Build history of the part. All positions in model axes, mm. A direction names the side the tool comes from. Give positions to 0.01 mm unless a question says otherwise; leave off trailing zeros. Loops run counter-clockwise (first coordinate to the right, second up) from the corner with the lowest first, then second, coordinate; pieces in that order, holes last.
1) Band-saw the part on B-B on x = -0.7. List the corners of the cut face in (y, z), then the cut area to 3 significant figures.
2) Band-saw the part on A-A on z = 0. List the corners of the cut face in (x, y).
3) Band-saw the part on D-D on x = 1.5. List the corners of the cut face in (y, z), then the cut area to 3 significant figures.
4) Two-plate mould, pull along X, no slides. Class faces 5 (the cylindrical face through (1, 6, 0)), 6 (the flat face through (-1.299, 1, 0)), 7 (the flat face through (1, 12, 1)): +X half, -X half, draft (parallel to the pull), parting line (faces both ways), or undercut.
5) Flat gauge pins, fed straight in: P1, Ø1.5, axis at y = 6.5, z = 1.5, coming from the -X side; P2, Ø1.6, axis at y = 1, z = 0, coming from the -X side; P3, Ø1.2, axis at y = 0.5, z = 0.5, coming from the +X side. Where does each tip first touch, or does it go through?
6) 3-axis set-ups, long thin cutter, end or side, ignore diameter. For faces 1 (the flat face through (1.299, 1, 0)), 2 (the flat face through (0.64, 0.99, -1.13)), 3 (the flat face through (-0.66, 0.99, -1.12)), 4 (the flat face through (0.66, 0.99, 1.12)): which of +Z, -Z, +X, -X, +Y, -Y reach the whole face in a straight line?
7) Wall check: line 1 (Z direction, x = 0, y = 6.25); line 2 (Y direction, x = -2.2, z = -0.2). Give the ranges that are in metal, low to high.
8) Band-saw the part on C-C on y = 4.5. List the corners of the cut face in (x, z), then the cut area to 3 significant figures.
Autodesk Inventor part; units mm, degrees
ref_plane "YZ Plane" through (0, 0, 0) normal (1, 0, 0) x (0, 1, 0)
ref_plane "XZ Plane" through (0, 0, 0) normal (0, 1, 0) x (-1, 0, 0)
ref_plane "XY Plane" through (0, 0, 0) normal (0, 0, 1) x (1, 0, 0)
sketch "Sketch1" plane through (0, 0, 0) normal (0, 1, 0) x (-1, 0, 0)
  circle A0 centre (0, 0) radius 1.5 construction
  line L0 (0, -1.5) -> (-1.299, -0.75)
  line L1 (-1.299, -0.75) -> (-1.299, 0.75)
  line L2 (-1.299, 0.75) -> (0, 1.5)
  line L3 (0, 1.5) -> (1.299, 0.75)
  line L4 (1.299, 0.75) -> (1.299, -0.75)
  line L5 (1.299, -0.75) -> (0, -1.5)
  dimension "d0" = 3
extrude "Extrusion1" add sketch "Sketch1" along normal blind 2
sketch "Sketch2" plane through (0, 2, 0) normal (0, 1, 0) x (1, 0, 0)
  circle A0 centre (0, 0) radius 2.5
  dimension "d3" = 5
extrude "Extrusion2" add sketch "Sketch2" along normal blind 10
sketch "Sketch3" plane through (0, 12, 0) normal (0, 1, 0) x (1, 0, 0)
  circle A0 centre (0, 0) radius 2.5
hole "Hole1" at (0, 12, 0) direction (0, -1, 0) diameter 2 end through all
properties part number "separator" material "PET Plastic"
Findings below:
1. outline: (0, -1.1) - (2, -1.1) - (2, -2.4) - (12, -2.4) - (12, -0.71) - (0, -0.71) - close; (0, 0.71) - (12, 0.71) - (12, 2.4) - (2, 2.4) - (2, 1.1) - (0, 1.1) - close
1. area: 35.2 mm2
2. outline: (-2.5, 2) - (-1.3, 2) - (-1.3, 0) - (-1, 0) - (-1, 12) - (-2.5, 12) - close; (1, 0) - (1.3, 0) - (1.3, 2) - (2.5, 2) - (2.5, 12) - (1, 12) - close
3. outline: (2, -2) - (12, -2) - (12, 2) - (2, 2) - close
3. area: 40.0 mm2
4. face 5: undercut
4. face 6: -X half
4. face 7: draft
5. P1: stops at x = -2.38
5. P2: stops at x = -1.3
5. P3: stops at x = 1.3
6. face 1: +Z, -Z, +X, -Y
6. face 2: -Z, +X, -Y
6. face 3: -Z, -X, -Y
6. face 4: +Z, +X, -Y
7. line 1: z = -2.5 to -1, 1 to 2.5
7. line 2: y = 2 to 12
8. outline: circle Ø5 at (0, 0); hole circle Ø2 at (0, 0)
8. area: 16.5 mm2
